Verification items for the finished model (mm, model axes). Face numbers are marked on the shaded views. A direction names the side the tool comes from. Coordinates: 2 decimals unless noted, no trailing zeros. Order: outer loops, then holes, each group sorted by start corner. A loop starts at its lowest first (then second) coordinate and runs counter-clockwise, first axis right, second up.
Q1. Cross-section at D-D, the plane z = 673. Record the boundary of the cut face in (x, y).
Q2. Depth check by flat-ended pin: P1, Ø9, axis at x = -413, z = 9, coming from the -Y side; P2, Ø1, axis at x = -177, y = 462.5, coming from the +Z side; P3, Ø18.5, axis at x = -387.5, y = 32.5, coming from the +Z side. Enter the tip coordinate at first touch or a pass-through.
Q3. Cross-section at C-C, the plane y = 205.5. Record the boundary of the cut face in (x, z).
Q4. Cross-section at A-A, the plane z = 197. Record the boundary of the cut face in (x, y), and give its area (3 significant figures).
Q5. Thickness scan on line 1 (X direction, y = 428.5, z = 239); line 2 (Z direction, x = -123.5, y = 366.5); line 3 (Y direction, x = -63, z = 660.5). Record the ranges inside material, lowest first.
Q6. Cross-section at B-B, the plane x = -229.5. Record the boundary of the cut face in (y, z).
Q7. Set-up check for the marked faces 4 and 5: record each of +Z, -Z, +X, -X, +Y, -Y from which the full face is reachable in a straight line by a thin tool's end or side.
Q8. Draft check along X on the marked faces 1, 2 and 3. Enter one of: pulls with the +X half, pulls with the -X half, needs draft (parallel to the pull), parting line crosses it, or undercut.
from build123d import *

# Parameters (mm, degrees)
F0_W      = 52.5068640709
F0_H      = 40.332518518
F1_DEPTH  = 560
F2_DEPTH  = 600
F3_DEPTH  = 720
F4_T      = -18
F5_W      = 27.2077894211
F5_H      = 138.2559251785
F6_DEPTH  = 562
F7_DEPTH  = 2
F8_W      = 16.7428851128
F8_H      = 76.9920415878
F9_DEPTH  = 564
F11_DEPTH = 10
F13_DEPTH = 10
F14_DEPTH = 16.5


with BuildPart() as f1:
    # F0 (on Front) → F1 (new body)
    with BuildSketch(Plane.XZ):
        with Locations((-26.2534320354, 20.166259259)):
            Rectangle(F0_W, F0_H)
    extrude(amount=-F1_DEPTH)

    # F2 (add): a face of the model
    f2_faces = [f1.faces().sort_by_distance(p)[0] for p in [
        (0, 280, 20.166259259),
    ]]
    extrude(f2_faces, amount=-F2_DEPTH)

    # F3 (add): a face of the model
    f3_faces = [f1.faces().sort_by_distance(p)[0] for p in [
        (-300, 280, 0),
    ]]
    extrude(f3_faces, amount=-F3_DEPTH)

    # F4
    f4_openings = [f1.faces().sort_by_distance(p)[0] for p in [
        (-300, 560, 360),
        (-300, 280, 720),
        (-300, 0, 360),
    ]]
    offset(amount=F4_T, openings=f4_openings)

    # F5 (on face) → F6 (join)
    with BuildSketch(Plane(origin=(-18, 0, 0), x_dir=(0, -1, 0), z_dir=(-1, 0, 0))):
        with Locations((-546.3961052895, 650.8720374107)):
            Rectangle(F5_W, F5_H)
    extrude(amount=F6_DEPTH)

    # F7 (add): a face of the model
    f7_faces = [f1.faces().sort_by_distance(p)[0] for p in [
        (-580, 546.3961052895, 650.8720374107),
    ]]
    extrude(f7_faces, amount=F7_DEPTH)

    # F8 (on face) → F9 (join)
    with BuildSketch(Plane(origin=(-18, 0, 0), x_dir=(0, -1, 0), z_dir=(-1, 0, 0))):
        with Locations((-34.7199738026, 56.4960207939)):
            Rectangle(F8_W, F8_H)
    extrude(amount=F9_DEPTH)

    # F10 (on face) → F11 (cut)
    with BuildSketch(Plane.XZ):
        Polygon((-18, 0), (-18, 18), (-582, 18), (-582, 720), (-600, 720), (-600, 0), align=None)
    extrude(amount=-F11_DEPTH, mode=Mode.SUBTRACT)

    # F12 (on face) → F13 (join)
    with BuildSketch(Plane.XZ.offset(-10)):
        Polygon((-582, 0), (-582, 18), (-582, 720), (-600, 720), (-600, 0), align=None)
    extrude(amount=F13_DEPTH)

    # F14 (cut): a face of the model
    f14_faces = [f1.faces().sort_by_distance(p)[0] for p in [
        (-300, 10, 9),
    ]]
    extrude(f14_faces, amount=-F14_DEPTH, mode=Mode.SUBTRACT)


solid = f1.part
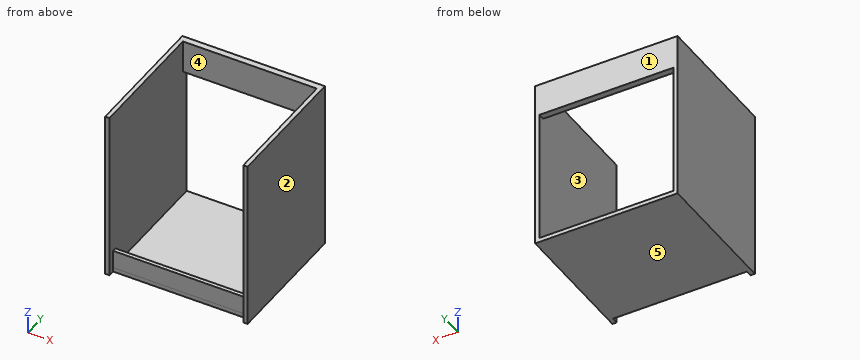
Check values:
1. outline: (-600, 0) - (-582, 0) - (-582, 532.79) - (-18, 532.79) - (-18, 0) - (0, 0) - (0, 560) - (-600, 560) - close
2. P1: stops at y = 26.5
2. P2: stops at z = 18
2. P3: stops at z = 94.99
3. outline: (-600, 0) - (0, 0) - (0, 720) - (-18, 720) - (-18, 18) - (-582, 18) - (-582, 720) - (-600, 720) - close
4. outline: (-600, 0) - (-582, 0) - (-582, 560) - (-600, 560) - close; (-18, 0) - (0, 0) - (0, 560) - (-18, 560) - close
4. area: 20,200 mm2
5. line 1: x = -600 to -582, -18 to 0
5. line 2: z = 0 to 18
5. line 3: y = 532.79 to 560
6. outline: (26.35, 18) - (26.5, 18) - (26.5, 0) - (560, 0) - (560, 18) - (43.09, 18) - (43.09, 94.99) - (26.35, 94.99) - close; (532.79, 581.74) - (560, 581.74) - (560, 720) - (532.79, 720) - close
7. face 4: +Z, -Y
7. face 5: -Z, +X, -X, +Y, -Y
8. face 1: needs draft
8. face 2: pulls with the +X half
8. face 3: undercut
